from build123d import *

# Parameters (mm, degrees)
F0_W      = 76.2
F0_H      = 177.8
F1_DEPTH  = 25.4
F1_FACE_W = 76.2
F1_FACE_H = 177.8
F2_DEPTH  = 25.4
F4_R      = 42.536427
F5_DEPTH  = 25.4
F5_FACE_R = 42.536427
F6_DEPTH  = 25.4


with BuildPart() as f1:
    # F0 (on Top) → F1 (new body)
    with BuildSketch(Plane.XY):
        with Locations((-12.912218, -4.254788)):
            Rectangle(F0_W, F0_H)
    extrude(amount=F1_DEPTH)

    # F1_face (on face) → F2 (join)
    with BuildSketch(Plane(origin=(-12.912218, -4.254788, 25.4), x_dir=(1, 0, 0), z_dir=(0, 0, 1))):
        Rectangle(F1_FACE_W, F1_FACE_H)
    extrude(amount=F2_DEPTH)

    # F4 (on face) → F5 (join)
    with BuildSketch(Plane.XY.offset(50.8)):
        with Locations((1.229391, -75.656846)):
            Circle(F4_R)
    extrude(amount=F5_DEPTH)

    # F5_face (on face) → F6 (join)
    with BuildSketch(Plane(origin=(1.229391, -75.656846, 76.2), x_dir=(1, 0, 0), z_dir=(0, 0, 1))):
        Circle(F5_FACE_R)
    extrude(amount=F6_DEPTH)


solid = f1.part
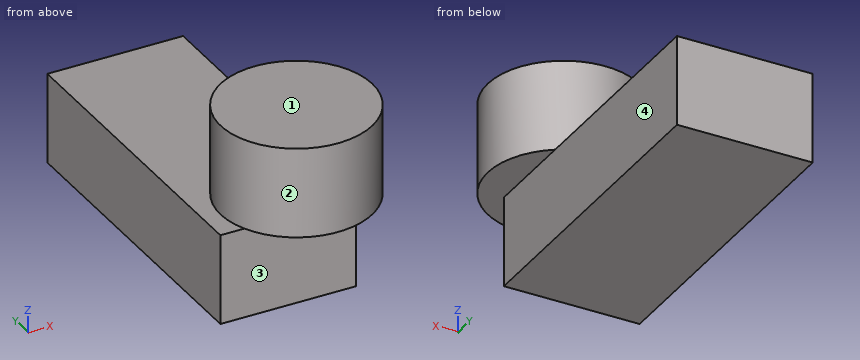
Work out the finished part from the listing and answer in its coordinate system (mm). Face numbers are marked on the shaded views. A direction names the side the tool comes from. Give positions to 0.01 mm unless a question says otherwise; leave off trailing zeros. Write each loop counter-clockwise with the first axis right and the second up, starting at its lowest first coordinate (ties: lowest second). Pieces come first, ordered by that corner, then holes.
Q1. A tool of negligible diameter and unlimited length cuts with its end or side. For the marked faces 1, 2, 3 and 4, from which of +Z, -Z, +X, -X, +Y, -Y can it reach the whole face along a straight path? Write none if from no direction.
Answer:
face 1: +Z, +X, -X, +Y, -Y
face 2: +Z
face 3: -Z, +X, -X, -Y
face 4: -Z, +X, +Y, -Y
Q2. The part is cut by section A-A on x = 0. Give the vertices of the cut face in (y, z).
Answer:
outline: (-118.18, 50.8) - (-93.15, 50.8) - (-93.15, 0) - (84.65, 0) - (84.65, 50.8) - (-33.14, 50.8) - (-33.14, 101.6) - (-118.18, 101.6) - close
Q3. The part is cut by section C-C on y = -85. Give the vertices of the cut face in (x, z), and give its area (3 significant figures).
Answer:
outline: (-51.01, 0) - (25.19, 0) - (25.19, 50.8) - (42.73, 50.8) - (42.73, 101.6) - (-40.27, 101.6) - (-40.27, 50.8) - (-51.01, 50.8) - close
area: 8,090 mm2
Q4. Given pin 1 (2 mm diameter, centred on x = -12.5, z = 35.5, fed in from -Y); pin 2 (2 mm diameter, centred on x = -22, z = 72, fed in from -Y); pin 3 (12 mm diameter, centred on x = -7, z = 69, fed in from -Y), each flat-ended and moving along its own axis, determine where each tip first touches the part or whether it passes through.
Answer:
pin 1: stops at y = -93.15
pin 2: stops at y = -111.92
pin 3: stops at y = -118.13
Q5. Straight lines are drawn through the part: L1, parallel to Z at x = 9.5, y = 29.5; L2, parallel to Z at x = 29, y = -47.5; L3, parallel to X at y = 39.5, z = 38. For each, find the intervals that lie inside material, in ascending order.
Answer:
L1: z = 0 to 50.8
L2: z = 50.8 to 101.6
L3: x = -51.01 to 25.19
Q6. The part is cut by section D-D on y = 5. Give the vertices of the cut face in (x, z), and give its area (3 significant figures).
Answer:
outline: (-51.01, 0) - (25.19, 0) - (25.19, 50.8) - (-51.01, 50.8) - close
area: 3,870 mm2
Q7. The part is cut by section B-B on z = 44. Give the vertices of the cut face in (x, y).
Answer:
outline: (-51.01, -93.15) - (25.19, -93.15) - (25.19, 84.65) - (-51.01, 84.65) - close
